For this review, use the dimensioned drawing (mm, ordinates from the lowest corner) and the shaded views. A direction names the side the tool comes from. Coordinates: 2 decimals unless noted, no trailing zeros. Loops run counter-clockwise (first coordinate to the right, second up) from the corner with the lowest first, then second, coordinate; pieces in that order, holes last. Notation, with made-up numbers: M -34.75,31.5 L 22.25,31.5 A20 cw 22.25,56.5 Z; hole C 50,12 d3. An arc over 180 degrees is marked long. One line per item, written item: value.
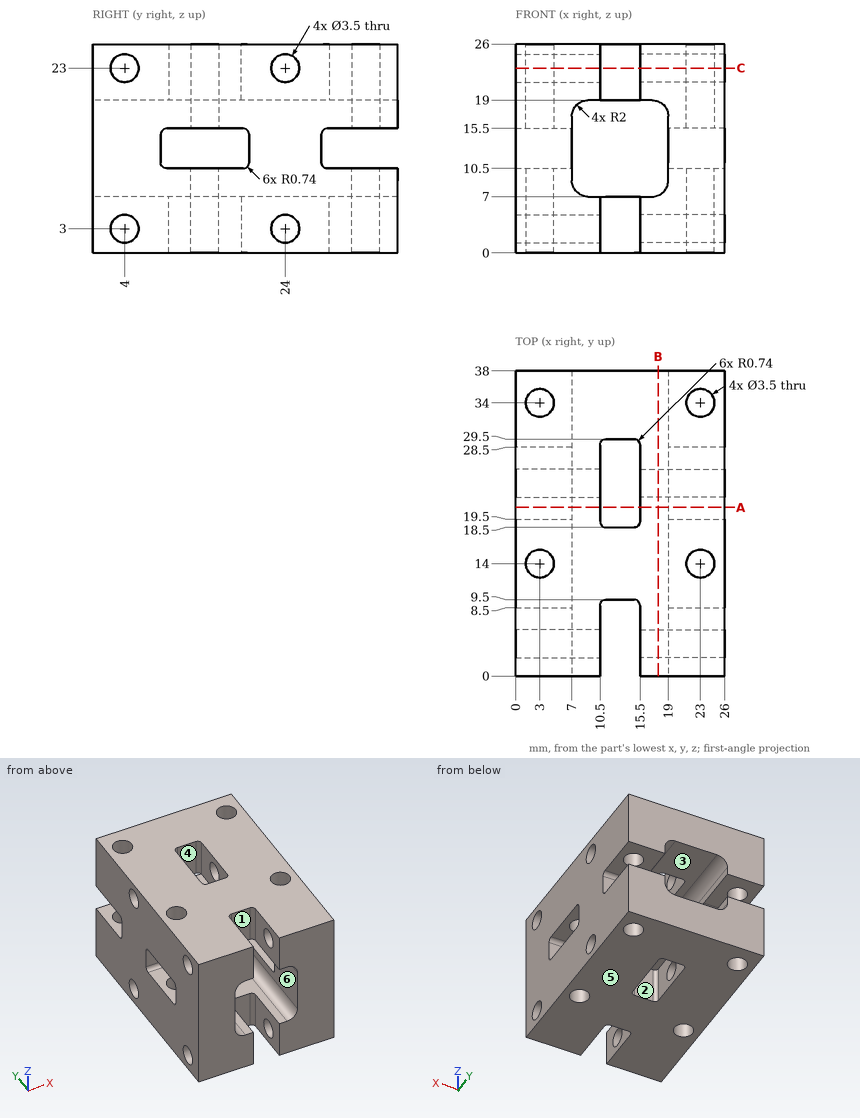
(1) We need section C-C on z = 23. State how many separate pieces and enclosed holes the cut face has, then the cut area to 3 significant figures.
Reply:
separate pieces: 4
enclosed holes: 4
area: 701 mm2
(2) We need section A-A on y = 21. State the section outline as (x, z) points, then the cut area to 3 significant figures.
Reply:
outline: M 0,0 L 10.5,0 L 10.5,7 L 9,7 A2 cw 7,9 L 7,17 A2 cw 9,19 L 10.5,19 L 10.5,26 L 0,26 Z; M 15.5,0 L 26,0 L 26,26 L 15.5,26 L 15.5,19 L 17,19 A2 cw 19,17 L 19,9 A2 cw 17,7 L 15.5,7 Z
area: 465 mm2
(3) Insertion check: pin 1 (4 mm diameter, centred on x = 13, z = 24, fed in from -Y). The pin has a flat end and moves straight along its axis. Give the tip position at first contact, or say it passes through.
Reply:
pin 1: stops at y = 9.46
(4) We need section B-B on x = 17.75. State the section outline as (y, z) points, then the cut area to 3 significant figures.
Reply:
outline: M 0,0 L 38,0 L 38,7.15 L 0,7.15 Z; M 0,18.85 L 38,18.85 L 38,26 L 0,26 Z; hole C 4,3 d3.5; hole C 4,23 d3.5; hole C 24,3 d3.5; hole C 24,23 d3.5
area: 505 mm2
(5) Mouldability with a two-part tool opening along Z and no side actions: class the marked faces 4, 5 and 6 as released by +Z, released by -Z, zero draft, split by the parting line, or undercut.
Reply:
face 4: zero draft
face 5: released by -Z
face 6: undercut
(6) To check wall thickness, follow line 1 along Y through (x, z) = (3, 7.25); line 2 along Z through (x, y) = (21, 4); line 3 along Z through (x, y) = (2.75, 17). State the ranges of each line that lie inside material, in increasing order. Write a range as [from, to].
Reply:
line 1: y = [0, 12.25], [15.75, 32.25], [35.75, 38]
line 2: z = [0, 1.25], [4.75, 21.25], [24.75, 26]
line 3: z = [0, 10.5], [15.5, 26]
(7) Tool access review of the marked faces 1, 2 and 3: name each direction out of +Z, -Z, +X, -X, +Y, -Y from which nothing blocks a thin tool from reaching the whole face with its end or side.
Reply:
face 1: +Z, -Z, -Y
face 2: +Z, -Z
face 3: +Y, -Y
